The listing builds one solid part. Answer for the finished solid, in the listing's coordinates (mm). Face numbers are marked on the shaded views. Coordinates: 2 decimals unless noted, no trailing zeros. Write each loop counter-clockwise with the first axis right and the second up, starting at its lowest first coordinate (ties: lowest second). Pieces come first, ordered by that corner, then holes.
from build123d import *

# Parameters (mm, degrees)
F0_W     = 38.1
F0_H     = 88.9
F1_DEPTH = 152.4
F3_D     = 12.7


# Not quite as in the source:
# - a feature of the source that left no trace in its solid (it failed there, or was rolled back) is left out
# - a length typed as a fraction of an inch, garbled in the dataset ("3 / 203.2 mm" for 3/8 in), is restored


with BuildPart() as f1:
    # F0 (on Right) → F1 (new body)
    with BuildSketch(Plane.YZ):
        Rectangle(F0_W, F0_H)
    extrude(amount=F1_DEPTH)

    # F3 (through all)
    with Locations(Plane.XZ.offset(19.05)):
        with Locations((76.2, 0)):
            Hole(F3_D / 2)


solid = f1.part
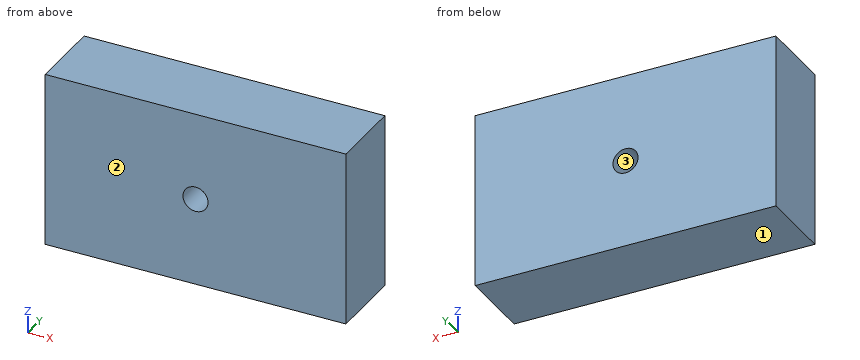
1. Section A-A on z = 0 is taken. Give the vertices of the cut face in (x, y), then the cut area to 3 significant figures.
Results found:
outline: (0, -19.05) - (69.85, -19.05) - (69.85, 19.05) - (0, 19.05) - close; (82.55, -19.05) - (152.4, -19.05) - (152.4, 19.05) - (82.55, 19.05) - close
area: 5,320 mm2
2. Find the intervals of material crossed by L1, parallel to Z at x = 76.2, y = 8.5; L2, parallel to Z at x = 75, y = 13, in increasing order.
Results found:
L1: z = -44.45 to -6.35, 6.35 to 44.45
L2: z = -44.45 to -6.24, 6.24 to 44.45
3. For a pull along Z with two mould halves and no side action, classify the marked faces 1, 2 and 3 as pulls with the +Z half, pulls with the -Z half, needs draft (parallel to the pull), parting line crosses it, or undercut.
Results found:
face 1: pulls with the -Z half
face 2: needs draft
face 3: undercut
4. Section B-B on x = 76.2 is taken. Give the vertices of the cut face in (y, z).
Results found:
outline: (-19.05, -44.45) - (19.05, -44.45) - (19.05, -6.35) - (-19.05, -6.35) - close; (-19.05, 6.35) - (19.05, 6.35) - (19.05, 44.45) - (-19.05, 44.45) - close
